```python
from build123d import *

# Parameters (mm, degrees)
BOSS_EXTRUDE1_DEPTH = 10
SKETCH2_R           = 6.5
SKETCH2_R_2         = 13
CUT_EXTRUDE1_DEPTH  = 10


with BuildPart() as part:
    # Sketch1 → Boss-Extrude1 (new body)
    with BuildSketch(Plane.XY):
        with BuildLine():
            Line((103.422242509, -51.995703566), (103.422242509, -82.995703566))
            Line((103.422242509, -82.995703566), (93.422242509, -92.995703566))
            Line((93.422242509, -92.995703566), (-8.05332169, -92.995703566))
            ThreePointArc((-8.05332169, -92.995703566), (-8.161516585, -92.963911368), (-8.235313944, -92.878642214))
            Line((-8.235313944, -92.878642214), (-94.615281586, 96.66489756))
            Line((-94.615281586, 96.66489756), (-89.662601304, 109.911442695))
            Line((-89.662601304, 109.911442695), (-62.363763178, 122.352239975))
            Line((-62.363763178, 122.352239975), (103.422242509, -51.995703566))
        make_face()
    extrude(amount=BOSS_EXTRUDE1_DEPTH)

    # Sketch2 → Cut-Extrude1 (cut)
    with BuildSketch(Plane.XY.offset(10)):
        with Locations((83.422242509, -68.995703566)):
            Circle(SKETCH2_R)
        with Locations((-64.03112347, 97.68108884)):
            Circle(SKETCH2_R)
        with Locations((-37.88844979, 57.424901579)):
            Circle(SKETCH2_R_2)
        with Locations((45.985961603, -71.730365885)):
            Circle(SKETCH2_R_2)
    extrude(amount=-CUT_EXTRUDE1_DEPTH, mode=Mode.SUBTRACT)


solid = part.part
```
CAD build for the part. Positions are in the model's coordinates, mm. Round coordinates to 2 decimals unless told otherwise and drop trailing zeros. Write each loop counter-clockwise with the first axis right and the second up, starting at its lowest first coordinate (ties: lowest second). Pieces come first, ordered by that corner, then holes. Notation, with made-up numbers: M -37.75,22 L -5.75,22 A17 cw -5.75,46 Z; hole C 2,12 d1. An arc over 180 degrees is marked long. One line per question, with ' | ' between items.
1. Probe L1, parallel to X at y = 69.5, z = 5.5; L2, parallel to Y at x = 41, z = 9; L3, parallel to X at y = 109, z = 8.25. List the from-to ranges inside material, lowest first. Write a range as from..to.
Working result:
L1: -82.24..-42.7, -33.07..-12.11 | L2: -93..-83.74, -59.72..13.65 | L3: -90..-49.67
2. Pin check, flat tips, straight feed: pin 1 Ø2 at (y, z) = (-1.5, 8) entering from -X; pin 2 Ø2 at (y, z) = (59.5, 1.5) entering from +X; pin 3 Ø1.5 at (y, z) = (98.5, 5.5) entering from -X. Stop position of each tip, or through.
Working result:
pin 1: x = -50.33 | pin 2: x = -1.65 | pin 3: x = -94.21
3. Mould opens along X. For faces 1 (the flat face through (-76.204, 116.045, 4.93)), 2 (the cylindrical face through (43.17, -84.42, 5.07)), 3 (the flat face through (6, -8, 0)) say: pulls with the +X half, pulls with the -X half, needs draft (parallel to the pull), parting line crosses it, or undercut.
Working result:
face 1: pulls with the -X half | face 2: undercut | face 3: needs draft
4. Cut at C-C on z = 7.5. Write the cut outline in (x, y).
Working result:
outline: M -94.62,96.66 L -8.24,-92.88 A0.2 ccw -8.05,-93 L 93.42,-93 L 103.42,-83 L 103.42,-52 L -62.36,122.35 L -89.66,109.91 Z; hole C -64.03,97.68 d13; hole C -37.89,57.42 d26; hole C 45.99,-71.73 d26; hole C 83.42,-69 d13
5. Cut at B-B on x = -36. Write the cut outline in (y, z).
Working result:
outline: M -31.95,0 L 44.56,0 L 44.56,10 L -31.95,10 Z; M 70.29,0 L 94.63,0 L 94.63,10 L 70.29,10 Z
6. Cut at D-D on y = -65.5. Write the cut outline in (x, z), and give its area (3 significant figures).
Working result:
outline: M -20.71,0 L 34.58,0 L 34.58,10 L -20.71,10 Z; M 57.4,0 L 77.94,0 L 77.94,10 L 57.4,10 Z; M 88.9,0 L 103.42,0 L 103.42,10 L 88.9,10 Z | area: 904 mm2
7. Cut at A-A on y = 54. Write the cut outline in (x, z).
Working result:
outline: M -75.17,0 L -50.43,0 L -50.43,10 L -75.17,10 Z; M -25.35,0 L 2.63,0 L 2.63,10 L -25.35,10 Z
